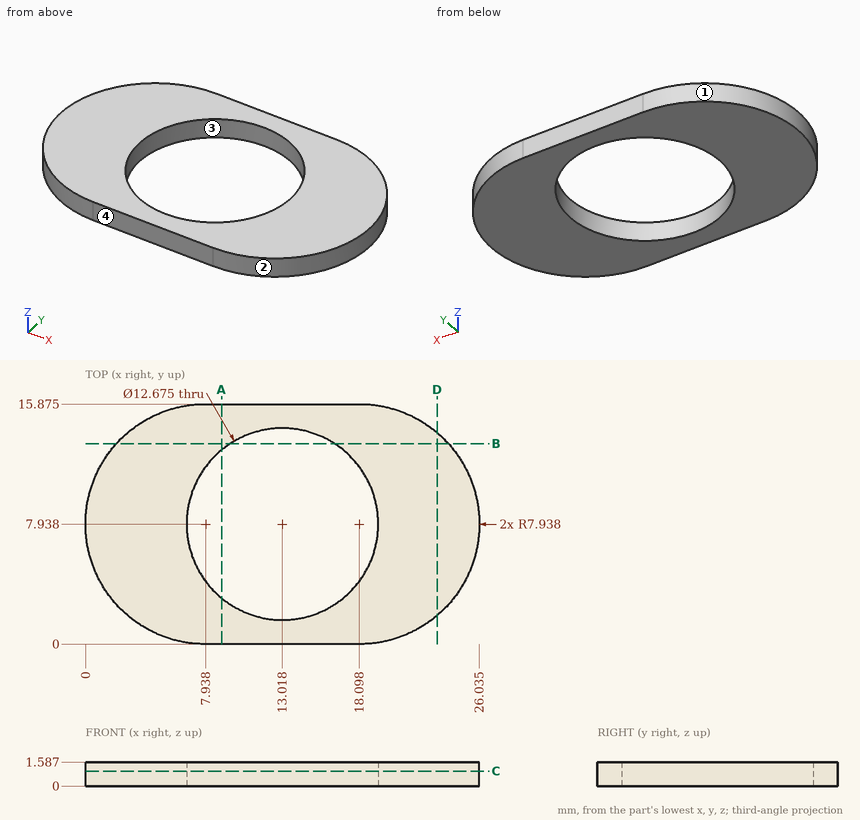
Design review of the part shown in the three views and the two pictorial views. Dimensions are in mm from the part's minimum x, y and z. Round coordinates to 2 decimals unless told otherwise and drop trailing zeros. Loops run counter-clockwise (first coordinate to the right, second up) from the corner with the lowest first, then second, coordinate; pieces in that order, holes last.
1) Consider section B-B on y = 13.25. State the section outline as (x, z) points (1 decimal).
Values follow:
outline: (2, 0) - (9.6, 0) - (9.6, 1.6) - (2, 1.6) - close; (16.5, 0) - (24, 0) - (24, 1.6) - (16.5, 1.6) - close
2) The part is to be moulded in two halves that separate along X. For the marked faces 1, 2, 3 and 4, say which applies: pulls with the +X half, pulls with the -X half, needs draft (parallel to the pull), parting line crosses it, or undercut.
Values follow:
face 1: pulls with the -X half
face 2: pulls with the +X half
face 3: undercut
face 4: needs draft
3) Consider section C-C on z = 1. State the section outline as (x, y) points (1 decimal), then the cut area to 3 significant figures.
Values follow:
outline: (7.9, 0) - (18.1, 0) arc R7.9 ccw to (18.1, 15.9) - (7.9, 15.9) arc R7.9 ccw to start; hole circle Ø12.7 at (13, 7.9)
area: 233 mm2
4) Consider section A-A on x = 9. State the section outline as (y, z) points (1 decimal).
Values follow:
outline: (0, 0) - (3, 0) - (3, 1.6) - (0, 1.6) - close; (12.8, 0) - (15.9, 0) - (15.9, 1.6) - (12.8, 1.6) - close
5) Wall thickness on line 1 along X through (y, z) = (12, 0.9) (1 decimal); line 2 along X through (y, z) = (9.75, 1.5) (1 decimal); line 3 along Y through (x, z) = (13.5, 0.5) (1 decimal): over which ranges is each line inside the solid? List them lowest first.
Values follow:
line 1: x = 1.1 to 8.2, 17.9 to 24.9
line 2: x = 0.2 to 6.9, 19.1 to 25.8
line 3: y = 0 to 1.6, 14.3 to 15.9
6) Consider section D-D on x = 23.25. State the section outline as (y, z) points (1 decimal).
Values follow:
outline: (1.9, 0) - (14, 0) - (14, 1.6) - (1.9, 1.6) - close
